from build123d import *

# Parameters (mm, degrees)
SKETCH_1_R               = 12.5
EXTRUDE_1_DEPTH          = 104
SKETCH_6_W               = 1
SKETCH_6_H               = 1.7
SKETCH_7_R               = 8
EXTRUDE_2_DEPTH          = 2
HOLE_WIZARD_M8_1_D       = 6.8
HOLE_WIZARD_M8_1_DEPTH   = 82.25
HOLE_WIZARD_M8_1_TIP     = 2.042926105
SKETCH_9_R               = 9
EXTRUDE_3_DEPTH          = 34
CUT_EXTRUDE_1_DEPTH      = 140.127639238
CUT_EXTRUDE_1_DEPTH_BACK = 140.127639238
SKETCH_8_W               = 34
SKETCH_8_H               = 10.443945465
CHAMFER_1_SIZE           = 3
HOLE_WIZARD_5_0_5_1_D    = 5
SKETCH_13_R              = 6
CUT_EXTRUDE_3_DEPTH      = 1


with BuildPart() as part:
    # 草图1 → 凸台-拉伸1 (new body)
    with BuildSketch(Plane.XY):
        with Locations(Location((0, 0, 0), (0, 0, 180))):
            Circle(SKETCH_1_R)
    extrude(amount=EXTRUDE_1_DEPTH)

    # 草图6 → 切除-旋转1 (revolve, cut)
    with BuildSketch(Plane(origin=(0, 0, 0), x_dir=(1, 0, 0), z_dir=(0, 1, 0))):
        with Locations((-12, -101.85)):
            Rectangle(SKETCH_6_W, SKETCH_6_H)
    revolve(axis=Axis((0, 0, 0), (0, 0, 1)), mode=Mode.SUBTRACT)

    # 草图7 → 凸台-拉伸2 (add)
    with BuildSketch(Plane(origin=(0, 0, 0), x_dir=(-1, 0, 0), z_dir=(0, 0, -1))):
        with Locations(Location((0, 0, 0), (0, 0, 180))):
            Circle(SKETCH_7_R)
    extrude(amount=EXTRUDE_2_DEPTH)

    # M8 螺纹孔1
    with Locations(Plane(origin=(0, 0, -2), x_dir=(-1, 0, 0), z_dir=(0, 0, -1))):
        with Locations((0, 0)):
            Hole(HOLE_WIZARD_M8_1_D / 2, depth=HOLE_WIZARD_M8_1_DEPTH)
            with Locations((0, 0, -(HOLE_WIZARD_M8_1_DEPTH + HOLE_WIZARD_M8_1_TIP / 2))):  # 118° drill point
                Cone(0, HOLE_WIZARD_M8_1_D / 2, HOLE_WIZARD_M8_1_TIP, mode=Mode.SUBTRACT)

    # 草图9 → 凸台-拉伸3 (add)
    with BuildSketch(Plane.XY.offset(104)):
        with Locations((-0.231058247, 0)):
            Circle(SKETCH_9_R)
    extrude(amount=EXTRUDE_3_DEPTH)

    # 草图8 → 切除-拉伸1 (cut, two sides: drawn at the far end of the back side and taken through both)
    with BuildSketch(Plane(origin=(0, 0, 0), x_dir=(0, 0, -1), z_dir=(0, 1, 0)).offset(-CUT_EXTRUDE_1_DEPTH_BACK)):
        with Locations((-121, 9.721972732)):
            Rectangle(SKETCH_8_W, SKETCH_8_H)
        with Locations((-121, -9.721972732)):
            Rectangle(SKETCH_8_W, SKETCH_8_H)
    extrude(amount=CUT_EXTRUDE_1_DEPTH + CUT_EXTRUDE_1_DEPTH_BACK, mode=Mode.SUBTRACT)

    # 倒角1
    chamfer_1_edges = [part.edges().sort_by_distance(p)[0] for p in [
        (0.035783968, -8.99604331, 138),
        (0.035783968, 8.99604331, 138),
    ]]
    chamfer(chamfer_1_edges, length=CHAMFER_1_SIZE)

    # Ø5.0 (5) 直径孔1 (through all)
    with Locations(Plane(origin=(4.5, 0, 0), x_dir=(0, 0, -1), z_dir=(1, 0, 0))):
        with Locations((-110, -3), (-134, 3)):
            Hole(HOLE_WIZARD_5_0_5_1_D / 2)

    # 草图13 → 切除-拉伸3 (cut)
    with BuildSketch(Plane(origin=(4.5, 0, 0), x_dir=(0, 0, -1), z_dir=(1, 0, 0))):
        with Locations((-134, 3)):
            Circle(SKETCH_13_R)
        with Locations((-110, -3)):
            Circle(SKETCH_13_R)
    cut_extrude_3 = extrude(amount=-CUT_EXTRUDE_3_DEPTH, mode=Mode.SUBTRACT)

    # 镜向1: 切除-拉伸3 across plane
    add(cut_extrude_3.mirror(Plane(origin=(0, 0, 0), x_dir=(0, 0, 1), z_dir=(1, 0, 0))), mode=Mode.SUBTRACT)


solid = part.part
Input: part model. Units: mm. Frame: model coordinates. A direction names the side the tool comes from. Give positions to 0.01 mm unless a question says otherwise; leave off trailing zeros. Write each loop counter-clockwise with the first axis right and the second up, starting at its lowest first coordinate (ties: lowest second). Pieces come first, ordered by that corner, then holes. Notation, with made-up numbers: (15, -7.5) -> (27, -7.5) arc R18 ccw to (27, 1.5) -> close; hole circle Ø2 at (69, 0). An arc over 180 degrees is marked (long way). Use one line per item in the form item = value. Start each with the question number.
1) Section query A-A on z = 110. Return the cut outline in (x, y), then the cut area to 3 significant figures.
2) Draft query along Z for faces 4 (the flat face through (0, 0, 138)), 5 (the flat face through (-4.5, 0, 121)), 6 (the flat face through (-11, 4, 101)). Return one class per face: pulls with the +Z half, pulls with the -Z half, needs draft (parallel to the pull), parting line crosses it, or undercut.
3) Set-up query: faces 1 (the cylindrical face through (-0.03, -8.998, 119.283)), 2 (the cylindrical face through (4, 3, 110)), 3 (the flat face through (-4.5, -7, 105)). Return all of +Z, -Z, +X, -X, +Y, -Y with unobstructed straight access to the full face (end or side cutting, diameter ignored); none if empty.
4) Pin query (flat end, axial travel): pin 1 (14 mm diameter, centred on y = 3, z = 134, fed in from +X); pin 2 (11 mm diameter, centred on y = -3, z = 110, fed in from -X); pin 3 (3 mm diameter, centred on x = -8.5, y = -5, fed in from +Z). Return the tip coordinate at first contact, or that it passes through.
5) Ray query, probe 1 along Z at (x, y) = (6.25, 0); probe 2 along X at (y, z) = (7, 120); probe 3 along X at (y, z) = (-3, 76.5). Return the intervals inside material, ascending. Write a range as from..to.
6) Section query D-D on z = 77.5. Return the cut outline in (x, y), then the cut area to 3 significant figures.
7) Section query B-B on x = 6.75. Return the cut outline in (y, z).
8) Section query C-C on z = 94. Return the cut outline in (x, y).
Outcome:
q1.outline = (-4.5, 3) -> (-3.5, 3) -> (-3.5, -0.5) -> (3.5, -0.5) -> (3.5, 3) -> (4.5, 3) -> (4.5, 7.66) arc R9 ccw to (-4.5, 7.92) -> close; (-3.5, -8.39) arc R9 ccw to (3.5, -8.19) -> (3.5, -5.5) -> (-3.5, -5.5) -> close
q1.area = 97.8 mm^2
q2.face_4 = pulls with the +Z half
q2.face_5 = needs draft
q2.face_6 = undercut
q3.face_1 = +Z, -Y
q3.face_2 = +X
q3.face_3 = +Z, -X, +Y, -Y
q4.pin_1 = 4.5
q4.pin_2 = -3.5
q4.pin_3 = 104
q5.probe_1 = -2..104
q5.probe_2 = -4.5..4.5
q5.probe_3 = -12.13..-1.6, 1.6..12.13
q6.outline = circle Ø25 at (0, 0); hole circle Ø6.8 at (0, 0)
q6.area = 455 mm^2
q7.outline = (-10.52, 0) -> (-4.29, 0) -> (-4.29, -2) -> (4.29, -2) -> (4.29, 0) -> (10.52, 0) -> (10.52, 101) -> (9.31, 101) -> (9.31, 102.7) -> (10.52, 102.7) -> (10.52, 104) -> (-10.52, 104) -> (-10.52, 102.7) -> (-9.31, 102.7) -> (-9.31, 101) -> (-10.52, 101) -> close
q8.outline = circle Ø25 at (0, 0)
